from build123d import *

# Parameters (mm, degrees)
SKETCH1_W                     = 25.4
SKETCH1_H                     = 25.4
BOSS_EXTRUDE1_DEPTH           = 25.4
SKETCH2_W                     = 15.875
SKETCH2_H                     = 15.875
CUT_EXTRUDE1_DEPTH            = 26.4
TAP_DRILL_FOR_4_40_TAP1_D     = 2.2606
TAP_DRILL_FOR_4_40_TAP1_DEPTH = 10.7188
TAP_DRILL_FOR_4_40_TAP1_TIP   = 0.679152758
F_3_8_0_375_DIAMETER_HOLE1_D  = 9.525
TAP_DRILL_FOR_3_48_TAP1_D     = 1.9939
TAP_DRILL_FOR_3_48_TAP1_DEPTH = 4.7625


with BuildPart() as part:
    # Sketch1 → Boss-Extrude1 (new body)
    with BuildSketch(Plane(origin=(0, 0, 0), x_dir=(1, 0, 0), z_dir=(0, 1, 0))):
        with Locations((12.7, 12.7)):
            Rectangle(SKETCH1_W, SKETCH1_H)
    extrude(amount=BOSS_EXTRUDE1_DEPTH)

    # Sketch2 → Cut-Extrude1 (cut, through all)
    with BuildSketch(Plane(origin=(0, 25.4, 0), x_dir=(1, 0, 0), z_dir=(0, 1, 0))):
        with Locations((12.7, 12.7)):
            Rectangle(SKETCH2_W, SKETCH2_H)
    extrude(amount=-CUT_EXTRUDE1_DEPTH, mode=Mode.SUBTRACT)

    # Tap Drill for #4-40 Tap1
    with Locations(Plane(origin=(0, 0, 0), x_dir=(-1, 0, 0), z_dir=(0, -1, 0))):
        with Locations((-2.54, 2.54), (-22.86, 2.54), (-22.86, 22.86), (-2.54, 22.86)):
            Hole(TAP_DRILL_FOR_4_40_TAP1_D / 2, depth=TAP_DRILL_FOR_4_40_TAP1_DEPTH)
            with Locations((0, 0, -(TAP_DRILL_FOR_4_40_TAP1_DEPTH + TAP_DRILL_FOR_4_40_TAP1_TIP / 2))):  # 118° drill point
                Cone(0, TAP_DRILL_FOR_4_40_TAP1_D / 2, TAP_DRILL_FOR_4_40_TAP1_TIP, mode=Mode.SUBTRACT)

    # 3/8 (0.375) Diameter Hole1 (through all)
    with Locations(Plane(origin=(25.4, 0, 0), x_dir=(0, 0, -1), z_dir=(1, 0, 0))):
        with Locations((12.7, 12.7)):
            Hole(F_3_8_0_375_DIAMETER_HOLE1_D / 2)

    # Tap Drill for #3-48 Tap1
    with Locations(Plane(origin=(25.4, 0, 0), x_dir=(0, 0, -1), z_dir=(1, 0, 0))):
        with Locations((12.7, 20.1422), (12.7, 5.2578)):
            Hole(TAP_DRILL_FOR_3_48_TAP1_D / 2, depth=TAP_DRILL_FOR_3_48_TAP1_DEPTH)


solid = part.part
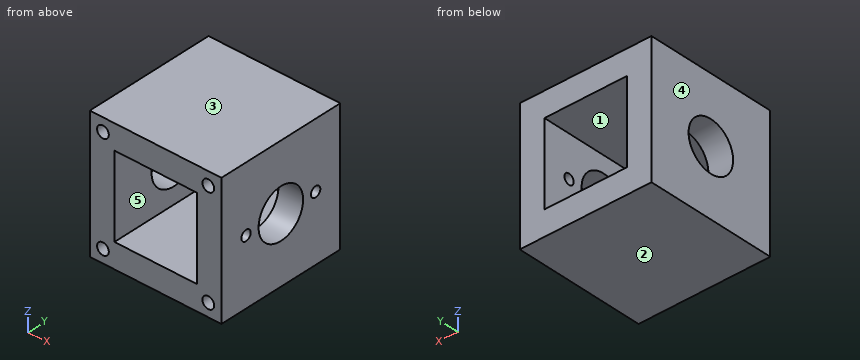
Source: CAD feature listing. Evaluate the final solid. Frame: model axes, mm. Face numbers are marked on the shaded views. A direction names the side the tool comes from. Give positions to 0.01 mm unless a question says otherwise; leave off trailing zeros. Loops run counter-clockwise (first coordinate to the right, second up) from the corner with the lowest first, then second, coordinate; pieces in that order, holes last. Notation, with made-up numbers: (-30.5, -8) -> (0.5, -8) arc R33 cw to (0.5, 26) -> close; hole circle Ø10 at (-19, 41). An arc over 180 degrees is marked (long way). Use a Markdown table: item, result. Add a question column.
1) Line query: line 1 along Y through (x, z) = (24.3, -12.7); line 2 along Z through (x, y) = (22.86, 6.5); line 3 along Z through (x, y) = (14.5, 18.5). Output: solid intervals per line, ascending. Write a range as [from, to].
2) Section query A-A, the plane z = -6. Return the cut outline in (x, y), then the cut area to 3 significant figures.
3) Pull-direction query (Z, two-part tool) for the marked faces 1, 2 and 3; classes: +Z half, -Z half, draft (parallel to the pull), parting line (faces both ways), or undercut.
4) Section query B-B, the plane y = 8.75. Return the cut outline in (x, z).
5) First-contact query: pin 1 (1.4 mm diameter, centred on x = 2.54, z = -2.54, fed in from -Y). Flat tip, straight axial feed; report the tip coordinate or a pass-through.
6) Reachability of the marked faces 4 and 5 from +Z, -Z, +X, -X, +Y, -Y: full face, straight path, thin tool, end or side. Return the list, or none.
7) Section query C-C, the plane x = 18.5. Return the cut outline in (y, z).
8) Section query D-D, the plane z = -12.7. Return the cut outline in (x, y), then the cut area to 3 significant figures.
Numbers:
| question | item | result |
|---|---|---|
| 1 | line 1 | y = [0, 4.26], [6.25, 7.94], [17.46, 19.15], [21.14, 25.4] |
| 1 | line 2 | z = [-25.4, -23.99], [-21.73, -3.67], [-1.41, 0] |
| 1 | line 3 | z = [-25.4, -20.64], [-4.76, 0] |
| 2 | outline | (0, 0) -> (4.76, 0) -> (4.76, 25.4) -> (0, 25.4) -> close; (20.64, 0) -> (25.4, 0) -> (25.4, 25.4) -> (20.64, 25.4) -> close |
| 2 | area | 242 mm2 |
| 3 | face 1 | undercut |
| 3 | face 2 | -Z half |
| 3 | face 3 | +Z half |
| 4 | outline | (0, -25.4) -> (25.4, -25.4) -> (25.4, -15.36) -> (20.64, -15.36) -> (20.64, -20.64) -> (4.76, -20.64) -> (4.76, -15.36) -> (0, -15.36) -> close; (0, -10.04) -> (4.76, -10.04) -> (4.76, -4.76) -> (20.64, -4.76) -> (20.64, -10.04) -> (25.4, -10.04) -> (25.4, 0) -> (0, 0) -> close; hole circle Ø2.26 at (2.54, -22.86); hole circle Ø2.26 at (2.54, -2.54); hole circle Ø2.26 at (22.86, -22.86); hole circle Ø2.26 at (22.86, -2.54) |
| 5 | pin 1 | stops at y = 10.98 |
| 6 | face 4 | +Z, -Z, -X, +Y, -Y |
| 6 | face 5 | +Y, -Y |
| 7 | outline | (0, -25.4) -> (25.4, -25.4) -> (25.4, -20.64) -> (0, -20.64) -> close; (0, -4.76) -> (25.4, -4.76) -> (25.4, 0) -> (0, 0) -> close |
| 8 | outline | (0, 0) -> (4.76, 0) -> (4.76, 7.94) -> (0, 7.94) -> close; (0, 17.46) -> (4.76, 17.46) -> (4.76, 25.4) -> (0, 25.4) -> close; (20.64, 0) -> (25.4, 0) -> (25.4, 4.26) -> (20.64, 4.26) -> close; (20.64, 6.25) -> (25.4, 6.25) -> (25.4, 7.94) -> (20.64, 7.94) -> close; (20.64, 17.46) -> (25.4, 17.46) -> (25.4, 19.15) -> (20.64, 19.15) -> close; (20.64, 21.14) -> (25.4, 21.14) -> (25.4, 25.4) -> (20.64, 25.4) -> close |
| 8 | area | 132 mm2 |
